```python
from build123d import *

# Parameters (mm, degrees)
SKETCH1_W               = 5
SKETCH1_H               = 163
BOSS_EXTRUDE1_DEPTH     = 3
BOSS_EXTRUDE2_DEPTH     = 81.5
BOSS_EXTRUDE3_START     = 81.5
BOSS_EXTRUDE3_DEPTH     = 81.5
SKETCH8_W               = 5
SKETCH8_H               = 10
BOSS_EXTRUDE4_DEPTH     = 3
SKETCH6_R               = 1.8
CUT_EXTRUDE1_DEPTH      = 92.58329542
SKETCH9_W               = 15
SKETCH9_H               = 163
BOSS_EXTRUDE5_DEPTH     = 3
FILLET1_R               = 1
CUT_EXTRUDE2_DEPTH      = 92.855865354
CUT_EXTRUDE2_DEPTH_BACK = 92.855865354
SKETCH10_R              = 1.8


with BuildPart() as part:
    # Sketch1 → Boss-Extrude1 (new body)
    with BuildSketch(Plane(origin=(0, 0, 0), x_dir=(1, 0, 0), z_dir=(0, 1, 0))):
        Rectangle(SKETCH1_W, SKETCH1_H)
    extrude(amount=BOSS_EXTRUDE1_DEPTH)

    # Sketch3 → Boss-Extrude2 (add)
    with BuildSketch(Plane.XY):
        with BuildLine():
            Line((-2.5, 3), (-2.5, 5.102989898))
            ThreePointArc((-2.5, 5.102989898), (0, 5.05), (2.5, 5.102989898))
            Line((2.5, 5.102989898), (2.5, 3))
            Line((2.5, 3), (2.5, 0))
            Line((2.5, 0), (-2.5, 0))
            Line((-2.5, 0), (-2.5, 3))
        make_face()
    extrude(amount=BOSS_EXTRUDE2_DEPTH)

    # Sketch7 → Boss-Extrude3 (add)
    with BuildSketch(Plane(origin=(0, 0, 0), x_dir=(-1, 0, 0), z_dir=(0, 0, -1)).offset(BOSS_EXTRUDE3_START)):
        with BuildLine():
            Line((-2.5, 5.102989898), (-2.5, 3))
            Line((-2.5, 3), (2.5, 3))
            Line((2.5, 3), (2.5, 5.102989898))
            ThreePointArc((2.5, 5.102989898), (0, 5.05), (-2.5, 5.102989898))
        make_face()
    extrude(amount=-BOSS_EXTRUDE3_DEPTH)

    # Sketch8 → Boss-Extrude4 (add)
    with BuildSketch(Plane.XZ):
        with Locations((0, 86.5)):
            Rectangle(SKETCH8_W, SKETCH8_H)
        with Locations((0, -86.5)):
            Rectangle(SKETCH8_W, SKETCH8_H)
    extrude(amount=-BOSS_EXTRUDE4_DEPTH)

    # Sketch6 → Cut-Extrude1 (cut, through all)
    with BuildSketch(Plane(origin=(0, 3, 0), x_dir=(1, 0, 0), z_dir=(0, 1, 0))):
        with Locations(Location((0, -88.5, 0), (0, 0, 270))):
            Circle(SKETCH6_R)
        with Locations(Location((0, 88.5, 0), (0, 0, 90))):
            Circle(SKETCH6_R)
    extrude(amount=-CUT_EXTRUDE1_DEPTH, mode=Mode.SUBTRACT)

    # Sketch9 → Boss-Extrude5 (add)
    with BuildSketch(Plane.XZ):
        Rectangle(SKETCH9_W, SKETCH9_H)
    extrude(amount=-BOSS_EXTRUDE5_DEPTH)

    # Fillet1
    # the kernel refuses this fillet: 1 mm, written as the material it adds along each edge
    with BuildSketch(Plane(origin=(2.5, 3, -81.5), x_dir=(0, 1, 0), z_dir=(0, 0, 1)), Plane(origin=(-2.5, 3, 81.5), x_dir=(0, 1, 0), z_dir=(0, 0, -1))) as fillet1_piece_1:
        with BuildLine():
            CenterArc((FILLET1_R, -FILLET1_R), FILLET1_R, 90, 90)
            Line((0, -FILLET1_R), (0, 0))
            Line((0, 0), (FILLET1_R, 0))
        make_face()
    extrude(amount=163)
    # the kernel refuses this fillet: 1 mm, written as the material it takes off along each edge
    with BuildSketch(Plane(origin=(-2.5, 5.102989898, 84.085592418), x_dir=(0, -1, 0), z_dir=(0, 0, -1))) as fillet1_2_piece_1:
        with BuildLine():
            CenterArc((1.034236967, -1), FILLET1_R, 90, 91.432543738)
            ThreePointArc((0.034549516, -1.025), (0.019501965, -0.512424928), (0, 0))
            Line((0, 0), (1.034236967, 0))
        make_face()
    extrude(amount=168.171184836, mode=Mode.SUBTRACT)
    with BuildSketch(Plane(origin=(2.5, 5.102989898, 84.085592418), x_dir=(0, -1, 0), z_dir=(0, 0, -1))) as fillet1_2_piece_2:
        with BuildLine():
            CenterArc((1.034236967, 1), FILLET1_R, 178.567456262, 91.432543738)
            ThreePointArc((0.034549516, 1.025), (0.019501965, 0.512424928), (0, 0))
            Line((0, 0), (1.034236967, 0))
        make_face()
    extrude(amount=168.171184836, mode=Mode.SUBTRACT)

    # Sketch10 → Cut-Extrude2 (cut, two sides: drawn at the far end of the back side and taken through both)
    with BuildSketch(Plane(origin=(0, 3, 0), x_dir=(1, 0, 0), z_dir=(0, 1, 0)).offset(-CUT_EXTRUDE2_DEPTH_BACK)):
        with Locations(Location((-3.75, -74, 0), (0, 0, 270))):
            Circle(SKETCH10_R)
        with Locations(Location((3.75, -68, 0), (0, 0, 270))):
            Circle(SKETCH10_R)
        with Locations(Location((3.75, 68, 0), (0, 0, 262.016443854))):
            Circle(SKETCH10_R)
        with Locations(Location((-3.75, 74, 0), (0, 0, 277.983556156))):
            Circle(SKETCH10_R)
    extrude(amount=CUT_EXTRUDE2_DEPTH + CUT_EXTRUDE2_DEPTH_BACK, mode=Mode.SUBTRACT)


solid = part.part
```
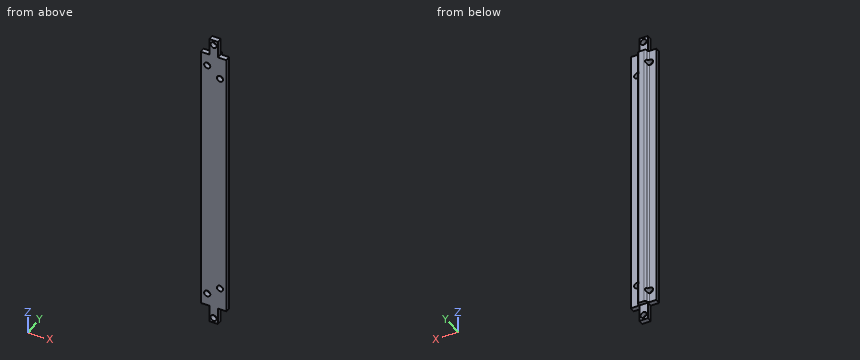
Input: part model. Units: mm. Frame: model coordinates. Round coordinates to 2 decimals unless told otherwise and drop trailing zeros. Loops run counter-clockwise (first coordinate to the right, second up) from the corner with the lowest first, then second, coordinate; pieces in that order, holes last. Notation, with made-up numbers: M 87.5,59.5 L 125.5,59.5 A31 cw 125.5,89.5 Z; hole C -28.5,44.25 d1. An arc over 180 degrees is marked long. Answer in a Markdown table with one row per item. Add a question column.
1. Contact query for flat-ended pins moving along their axis: pin 1 (2 mm diameter, centred on x = -5.5, z = 13, fed in from +Y); pin 2 (0.9 mm diameter, centred on y = 1, z = 88.5, fed in from -X); pin 3 (3 mm diameter, centred on x = 6, y = 4, fed in from +Z). Output: stop coordinate, or through.
2. Ray query, probe 1 along Z at (x, y) = (5, 1.35); probe 2 along X at (y, z) = (2.5, 74); probe 3 along X at (y, z) = (0.85, 88.5). Return the intervals inside material, ascending.
3. Section A-A (z = -88.5). Output: boundary loops of the cut face in (x, y), and give its area (3 significant figures).
4. Section B-B (y = 2.1). Output: boundary loops of the cut face in (x, z).
5. Section C-C (z = 2.5). Output: boundary loops of the cut face in (x, y) (3 decimals).
Values follow:
| question | item | result |
|---|---|---|
| 1 | pin 1 | y = 3 |
| 1 | pin 2 | x = -2.5 |
| 1 | pin 3 | z = 81.5 |
| 2 | probe 1 | -81.5 to -69.3, -66.7 to 66.7, 69.3 to 81.5 |
| 2 | probe 2 | -7.5 to -5.55, -1.95 to 7.5 |
| 2 | probe 3 | -2.5 to -1.8, 1.8 to 2.5 |
| 3 | outline | M -2.5,0 L -1.8,0 L -1.8,3 L -2.5,3 Z; M 1.8,0 L 2.5,0 L 2.5,3 L 1.8,3 Z |
| 3 | area | 4.20 mm^2 |
| 4 | outline | M -7.5,-81.5 L -2.5,-81.5 L -2.5,-91.5 L 2.5,-91.5 L 2.5,-81.5 L 7.5,-81.5 L 7.5,81.5 L 2.5,81.5 L 2.5,91.5 L -2.5,91.5 L -2.5,81.5 L -7.5,81.5 Z; hole C -3.75,-74 d3.6; hole C -3.75,74 d3.6; hole C 0,-88.5 d3.6; hole C 0,88.5 d3.6; hole C 3.75,-68 d3.6; hole C 3.75,68 d3.6 |
| 5 | outline | M -7.5,0 L 7.5,0 L 7.5,3 L 3.5,3 A1 cw 2.5,4 L 2.5,4.069 A1 ccw 1.475,5.068 A59 cw -1.475,5.068 A1 ccw -2.5,4.069 L -2.5,4 A1 cw -3.5,3 L -7.5,3 Z |
